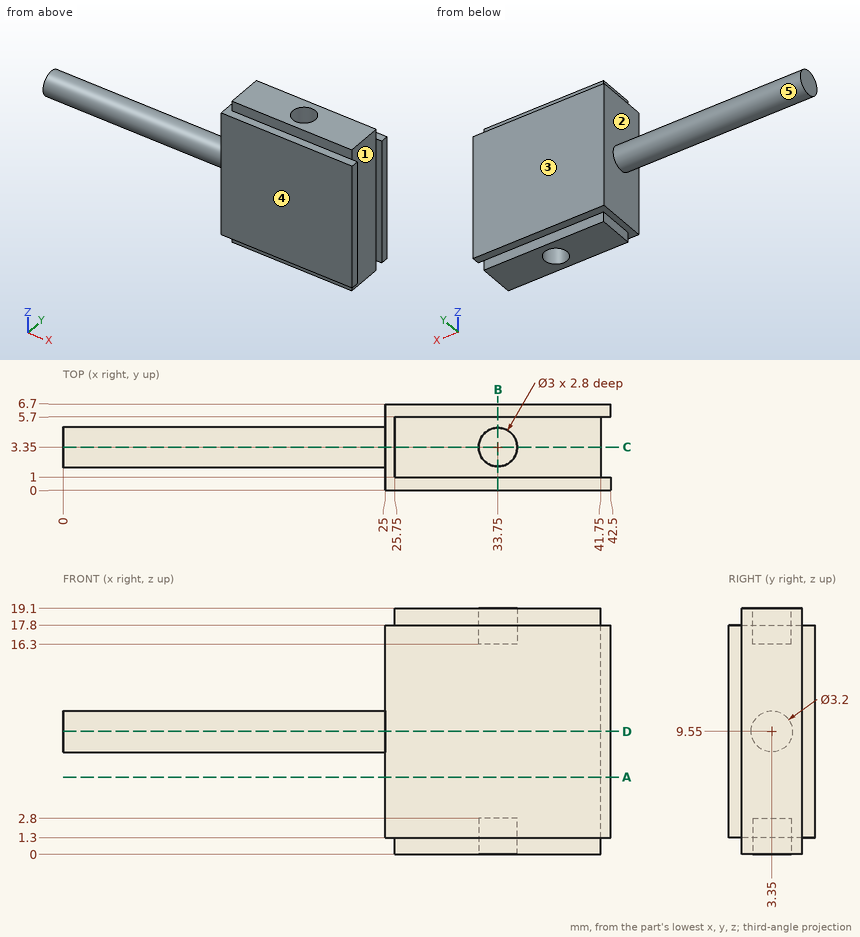
Study the drawing (mm; zero at the part's minimum x, y, z) and answer. A direction names the side the tool comes from. Coordinates: 2 decimals unless noted, no trailing zeros. Write each loop counter-clockwise with the first axis right and the second up, starting at its lowest first coordinate (ties: lowest second). Pieces come first, ordered by that corner, then holes. Notation, with made-up numbers: (-25, 19) - (14, 19) arc R14 ccw to (14, 24) - close; hole circle Ø10 at (-8, 6.25). An arc over 180 degrees is marked (long way). One line per question, with ' | ' between items.
1) The mould has two halves that part along Y. Classify the marked faces 1, 2 and 3: +Y half, -Y half, draft (parallel to the pull), parting line (faces both ways), or undercut.
Checks:
face 1: undercut | face 2: draft | face 3: +Y half
2) Find section C-C, the plane y = 3.35. Determine the outline of the cut face in (x, z), and give its area (3 significant figures).
Checks:
outline: (0, 7.95) - (25, 7.95) - (25, 1.3) - (25.75, 1.3) - (25.75, 0) - (32.25, 0) - (32.25, 2.8) - (35.25, 2.8) - (35.25, 0) - (41.75, 0) - (41.75, 19.1) - (35.25, 19.1) - (35.25, 16.3) - (32.25, 16.3) - (32.25, 19.1) - (25.75, 19.1) - (25.75, 17.8) - (25, 17.8) - (25, 11.15) - (0, 11.15) - close | area: 381 mm2
3) Find section A-A, the plane z = 6. Determine the outline of the cut face in (x, y), and give its area (3 significant figures).
Checks:
outline: (25, 0) - (42.5, 0) - (42.5, 1) - (41.75, 1) - (41.75, 5.7) - (42.5, 5.7) - (42.5, 6.7) - (25, 6.7) - close | area: 114 mm2
4) Flat-ended cylindrical pins translate along their axes: P1, Ø0.7, axis at x = 35.5, z = 1, coming from the +Y side; P2, Ø1.5, axis at x = 33.5, y = 3.5, coming from the +Z side; P3, Ø4, axis at y = 3.5, z = 9, coming from the +X side; P4, Ø1, axis at x = 30, z = 0.5, coming from the -Y side. Find the tip coordinate at first contact, or state that the pin passes through.
Checks:
P1: y = 6.7 | P2: z = 16.3 | P3: x = 41.75 | P4: y = 1
5) Find section B-B, the plane x = 33.75. Determine the outline of the cut face in (y, z).
Checks:
outline: (0, 1.3) - (1, 1.3) - (1, 0) - (1.85, 0) - (1.85, 2.8) - (4.85, 2.8) - (4.85, 0) - (5.7, 0) - (5.7, 1.3) - (6.7, 1.3) - (6.7, 17.8) - (5.7, 17.8) - (5.7, 19.1) - (4.85, 19.1) - (4.85, 16.3) - (1.85, 16.3) - (1.85, 19.1) - (1, 19.1) - (1, 17.8) - (0, 17.8) - close
6) For the marked faces 4 and 5, determine the directions among +Z, -Z, +X, -X, +Y, -Y from which every point of the face is accessible in a straight line to the end or side of a thin tool.
Checks:
face 4: +Z, -Z, +X, -X, -Y | face 5: -X
7) Find section D-D, the plane z = 9.55. Determine the outline of the cut face in (x, y).
Checks:
outline: (0, 1.75) - (25, 1.75) - (25, 0) - (42.5, 0) - (42.5, 1) - (41.75, 1) - (41.75, 5.7) - (42.5, 5.7) - (42.5, 6.7) - (25, 6.7) - (25, 4.95) - (0, 4.95) - close
8) Consider probe 1 along Y at (x, z) = (33.75, 17.85); probe 2 along X at (y, z) = (3.35, 1.1); probe 3 along Y at (x, z) = (33.75, 2.1). Determine where each line is inside the solid, lowest interval first. Write a range as [from, to].
Checks:
probe 1: [1, 1.85], [4.85, 5.7] | probe 2: [25.75, 32.25], [35.25, 41.75] | probe 3: [0, 1.85], [4.85, 6.7]
